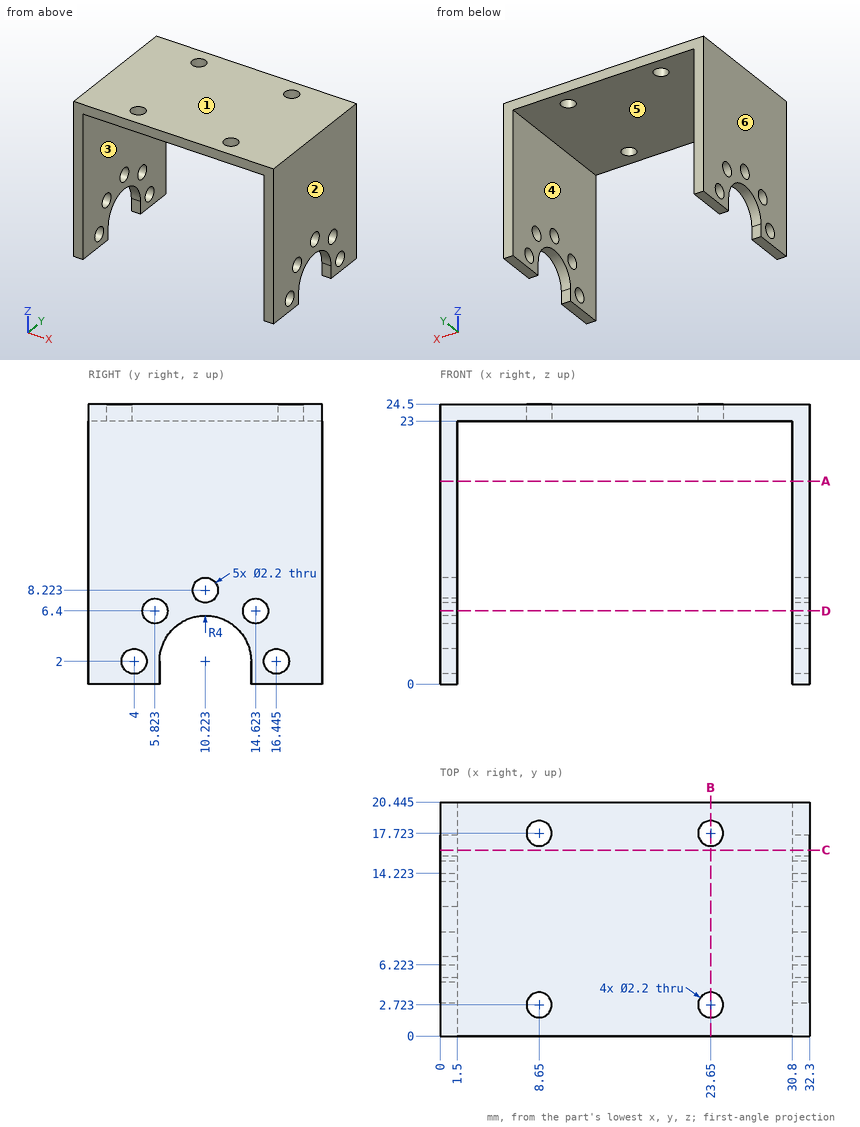
Drawing for the job (mm, zero at the part's lowest x, y, z). A direction names the side the tool comes from. Round coordinates to 2 decimals unless told otherwise and drop trailing zeros. Loops run counter-clockwise (first coordinate to the right, second up) from the corner with the lowest first, then second, coordinate; pieces in that order, holes last. Notation, with made-up numbers: (30, 61.25) - (65, 61.25) arc R13 cw to (65, 70.25) - close; hole circle Ø3 at (84, -11). An arc over 180 degrees is marked (long way). Write each question's results on one line, items separated by ' | '.
(1) Saw through at A-A, the plane z = 17.75. List the corners of the cut face in (x, y) (1 decimal).
Answer below:
outline: (0, 0) - (1.5, 0) - (1.5, 20.4) - (0, 20.4) - close; (30.8, 0) - (32.3, 0) - (32.3, 20.4) - (30.8, 20.4) - close
(2) 3-axis set-ups, long thin cutter, end or side, ignore diameter. For the marked faces 5 and 6: which of +Z, -Z, +X, -X, +Y, -Y reach the whole face in a straight line?
Answer below:
face 5: -Z, +Y, -Y | face 6: +Z, -Z, -X, +Y, -Y
(3) Mould opens along X. For the marked faces 1, 2, 3 and 4 say: released by +X, released by -X, zero draft, split by the parting line, or undercut.
Answer below:
face 1: zero draft | face 2: released by +X | face 3: undercut | face 4: undercut
(4) Pin check, flat tip, straight feed: pin 1 (3 mm diameter, centred on x = 23.65, y = 17.72, fed in from -Z). Stop position of the tip, or through.
Answer below:
pin 1: stops at z = 23
(5) Wall check: L1, parallel to Y at x = 23.65, z = 23.4 (1 decimal); L2, parallel to X at y = 17.5, z = 10.25; L3, parallel to Z at x = 0.9, y = 4. Give the ranges that are in metal, low to high.
Answer below:
L1: y = 0 to 1.6, 3.8 to 16.6, 18.8 to 20.4 | L2: x = 0 to 1.5, 30.8 to 32.3 | L3: z = 0 to 0.9, 3.1 to 24.5
(6) Saw through at B-B, the plane x = 23.65. List the corners of the cut face in (y, z) (1 decimal).
Answer below:
outline: (0, 23) - (1.6, 23) - (1.6, 24.5) - (0, 24.5) - close; (3.8, 23) - (16.6, 23) - (16.6, 24.5) - (3.8, 24.5) - close; (18.8, 23) - (20.4, 23) - (20.4, 24.5) - (18.8, 24.5) - close
(7) Saw through at D-D, the plane z = 6.4. List the corners of the cut face in (x, y) (1 decimal).
Answer below:
outline: (0, 0) - (1.5, 0) - (1.5, 4.7) - (0, 4.7) - close; (0, 6.9) - (1.5, 6.9) - (1.5, 13.5) - (0, 13.5) - close; (0, 15.7) - (1.5, 15.7) - (1.5, 20.4) - (0, 20.4) - close; (30.8, 0) - (32.3, 0) - (32.3, 4.7) - (30.8, 4.7) - close; (30.8, 6.9) - (32.3, 6.9) - (32.3, 13.5) - (30.8, 13.5) - close; (30.8, 15.7) - (32.3, 15.7) - (32.3, 20.4) - (30.8, 20.4) - close
(8) Saw through at C-C, the plane y = 16.25. List the corners of the cut face in (x, z), then the cut area to 3 significant figures.
Answer below:
outline: (0, 0) - (1.5, 0) - (1.5, 0.92) - (0, 0.92) - close; (0, 3.08) - (1.5, 3.08) - (1.5, 23) - (30.8, 23) - (30.8, 3.08) - (32.3, 3.08) - (32.3, 24.5) - (0, 24.5) - close; (30.8, 0) - (32.3, 0) - (32.3, 0.92) - (30.8, 0.92) - close | area: 111 mm^2
